Part model, mm, in its own coordinate system. Face numbers are marked on the shaded views. A direction names the side the tool comes from. Round coordinates to 2 decimals unless told otherwise and drop trailing zeros. Write each loop counter-clockwise with the first axis right and the second up, starting at its lowest first coordinate (ties: lowest second). Pieces come first, ordered by that corner, then holes. Notation, with made-up numbers: (71, 23) -> (80, 23) arc R20 cw to (80, 60) -> close; hole circle Ø11 at (19.5, 51.25). An arc over 180 degrees is marked (long way). Return JSON: item names as keys, results as strings. Group by question number.
(1) Saw through at C-C (z = -23.5). List the corners of the cut face in (x, y) (3 decimals), plus the area to 3 significant figures.
(2) Tool access for the marked faces 1 and 2: list every direction of +Z, -Z, +X, -X, +Y, -Y with a clear straight run to the whole face (end or side of a thin tool).
(3) Saw through at A-A (x = -2). State how many separate pieces and enclosed holes the cut face has, plus the area to 3 significant figures.
(4) Drill centre lines: L1, parallel to Z at x = 1.75, y = -1.75 (3 decimals); L2, parallel to Z at x = 1.5, y = 1.25 (3 decimals); L3, parallel to Y at x = 1, z = -30. Where is each one in solid material? Low to high. Write a range as from..to.
(5) Drop flat-ended pins along their axis: pin 1 Ø1.9 at (x, z) = (-0.5, -30) entering from +Y; pin 2 Ø1 at (x, y) = (-1.5, 9) entering from +Z; pin 3 Ø4 at (y, z) = (0, 15.875) entering from -X. Give the stop position or say it passes through.
(6) Saw through at B-B (y = 5.5). List the corners of the cut face in (x, z) (3 decimals).
(7) Saw through at D-D (y = 1.75). List the corners of the cut face in (x, z) (3 decimals).
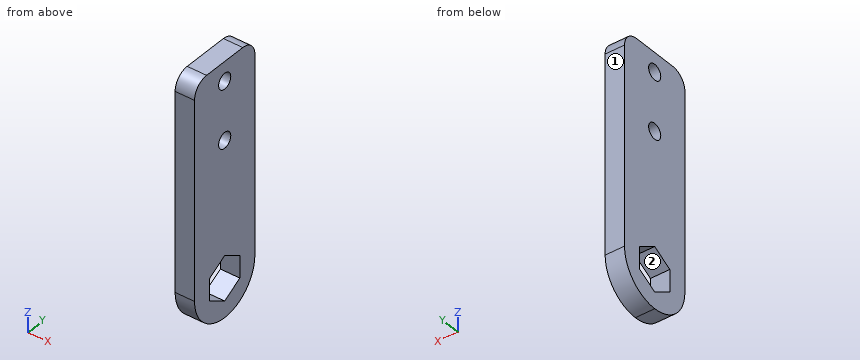
from build123d import *

# Parameters (mm, degrees)
SKETCH1_W              = 82.55
SKETCH1_H              = 25.4
BOSS_EXTRUDE1_DEPTH    = 3.175
FILLET1_R              = 12.7
F_10_CLEARANCE_HOLE1_D = 5.1054
FILLET2_R              = 5.08
CUT_EXTRUDE1_DEPTH     = 44.649033494


with BuildPart() as part:
    # Sketch1 → Boss-Extrude1 (new, symmetric)
    with BuildSketch(Plane(origin=(0, 0, 0), x_dir=(0, 0, -1), z_dir=(1, 0, 0))):
        Rectangle(SKETCH1_W, SKETCH1_H)
    extrude(amount=BOSS_EXTRUDE1_DEPTH, both=True)

    # Fillet1
    fillet1_edges = [part.edges().sort_by_distance(p)[0] for p in [
        (0, -12.7, -41.275),
        (0, 12.7, -41.275),
    ]]
    fillet(fillet1_edges, radius=FILLET1_R - 0.0001)  # a hair under: the kernel refuses the full size

    # #10 Clearance Hole1 (through all)
    with Locations(Plane(origin=(3.175, 6.272913445, 168.827028559), x_dir=(0, 0, -1), z_dir=(1, 0, 0))):
        with Locations((152.952028559, -6.272913445), (133.902028559, -6.272913445)):
            Hole(F_10_CLEARANCE_HOLE1_D / 2)

    # Fillet2
    fillet2_edges = [part.edges().sort_by_distance(p)[0] for p in [
        (0, -12.7, 41.275),
        (0, 12.7, 41.275),
    ]]
    fillet(fillet2_edges, radius=FILLET2_R)

    # Sketch7 → Cut-Extrude1 (cut, through all)
    with BuildSketch(Plane(origin=(3.175, 0, 0), x_dir=(0, 0, -1), z_dir=(1, 0, 0))):
        Polygon((32.241174209, 6.35), (24.908825791, 6.35), (21.242651581, 0), (24.908825791, -6.35), (32.241174209, -6.35), (35.907348419, 0), align=None)
    extrude(amount=-CUT_EXTRUDE1_DEPTH, mode=Mode.SUBTRACT)


solid = part.part
Computed values:
{
 "1": {"outline": "(-3.175, -12.7) -> (3.175, -12.7) -> (3.175, -3.91) -> (-3.175, -3.91) -> close; (-3.175, 3.91) -> (3.175, 3.91) -> (3.175, 12.7) -> (-3.175, 12.7) -> close", "area": "112 mm2"},
 "2": {"face 1": "+Z, -Z, +X, -X, +Y", "face 2": "+X, -X"},
 "3": {"separate pieces": "1", "enclosed holes": "3", "area": "1,840 mm2"},
 "4": {"L1": "-41.154..-34.897, -22.253..14.017, 17.733..33.067, 36.783..41.275", "L2": "-41.213..-35.186, -21.964..13.649, 18.101..32.699, 37.151..41.275", "L3": "-12.62..-6.35, 6.35..12.62"},
 "5": {"pin 1": "y = 12.69", "pin 2": "z = 41.2", "pin 3": "through"},
 "6": {"outline": "(-3.175, -40.022) -> (3.175, -40.022) -> (3.175, -32.732) -> (-3.175, -32.732) -> close; (-3.175, -24.418) -> (3.175, -24.418) -> (3.175, 41.275) -> (-3.175, 41.275) -> close"},
 "7": {"outline": "(-3.175, -41.154) -> (3.175, -41.154) -> (3.175, -34.897) -> (-3.175, -34.897) -> close; (-3.175, -22.253) -> (3.175, -22.253) -> (3.175, 14.017) -> (-3.175, 14.017) -> close; (-3.175, 17.733) -> (3.175, 17.733) -> (3.175, 33.067) -> (-3.175, 33.067) -> close; (-3.175, 36.783) -> (3.175, 36.783) -> (3.175, 41.275) -> (-3.175, 41.275) -> close"}
}
